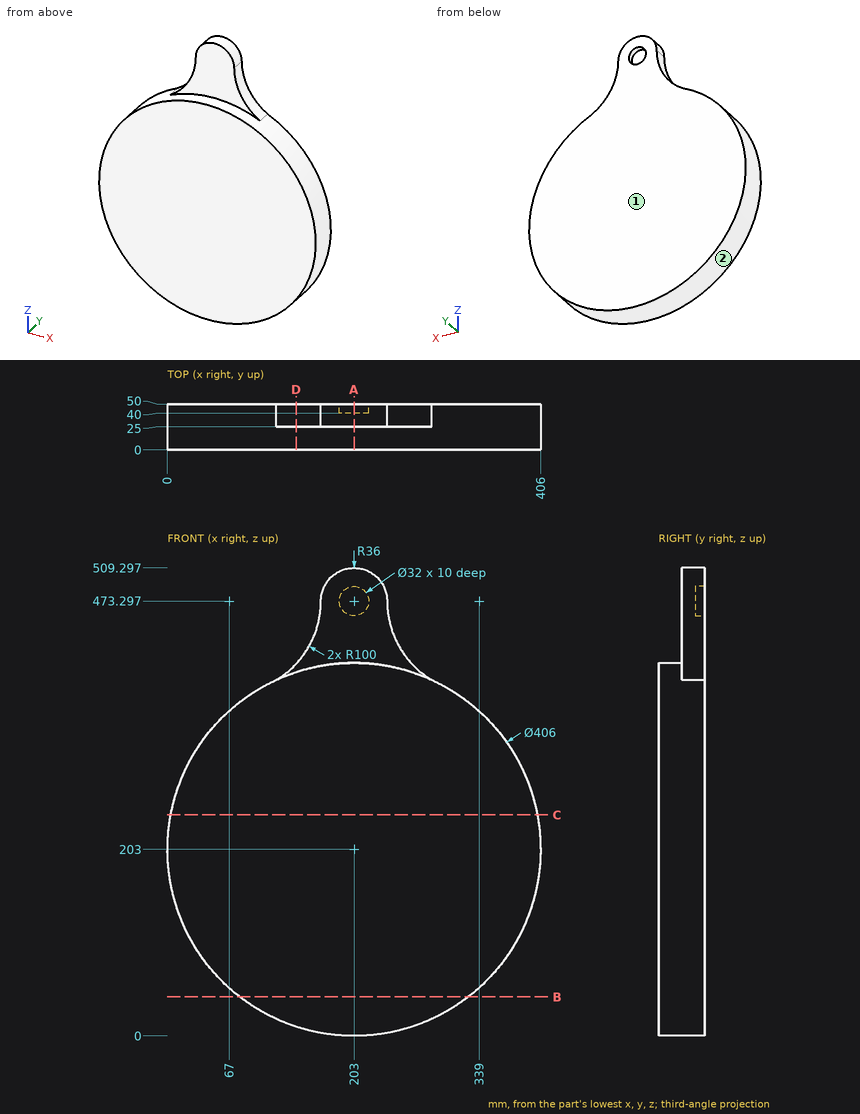
Drawing for the job (mm, zero at the part's lowest x, y, z). A direction names the side the tool comes from. Round coordinates to 2 decimals unless told otherwise and drop trailing zeros. Order: outer loops, then holes, each group sorted by start corner. A loop starts at its lowest first (then second) coordinate and runs counter-clockwise, first axis right, second up. Notation, with made-up numbers: (32.25, -16) -> (63.25, -16) arc R9 cw to (63.25, -2) -> close; hole circle Ø4 at (-1, 23). An arc over 180 degrees is marked (long way). Write item = value, one per line. Start each with the question number.
(1) Cut at C-C, the plane z = 240.5. List the corners of the cut face in (x, y).
(2) Cut at A-A, the plane x = 203. List the corners of the cut face in (y, z).
(3) Cut at B-B, the plane z = 42.5. List the corners of the cut face in (x, y).
(4) Cut at D-D, the plane x = 140. List the corners of the cut face in (y, z).
(5) Probe line 1 (X direction, y = 45, z = 206); line 2 (Y direction, x = 233.5, z = 411); line 3 (X direction, y = 4, z = 302). List the from-to ranges inside material, lowest first. Write a range as [from, to].
(6) Which spindle directions (+Z, -Z, +X, -X, +Y, -Y) get a long thin tool onto all of the face, cutting with end or side? Do the marked faces 1 and 2. Say none if no direction does.
(7) Pin check, flat tips, straight feed: P1, Ø1, axis at y = 18.5, z = 259, coming from the -X side; P2, Ø4, axis at y = 34, z = 437, coming from the -X side; P3, Ø5, axis at y = 29.5, z = 303.5, coming from the -X side. Stop position of each tip, or through.
Model answer:
q1.outline = (3.49, 0) -> (402.51, 0) -> (402.51, 50) -> (3.49, 50) -> close
q2.outline = (0, 0) -> (50, 0) -> (50, 457.3) -> (40, 457.3) -> (40, 489.3) -> (50, 489.3) -> (50, 509.3) -> (25, 509.3) -> (25, 406) -> (0, 406) -> close
q3.outline = (78.71, 0) -> (327.29, 0) -> (327.29, 50) -> (78.71, 50) -> close
q4.outline = (0, 10.02) -> (50, 10.02) -> (50, 404.95) -> (25, 404.95) -> (25, 395.98) -> (0, 395.98) -> close
q5.line_1 = [0.02, 405.98]
q5.line_2 = [25, 50]
q5.line_3 = [25.78, 380.22]
q6.face_1 = +Z, -Z, +X, -X, +Y
q6.face_2 = -Y
q7.P1 = 7.73
q7.P2 = 159.38
q7.P3 = 25.22
